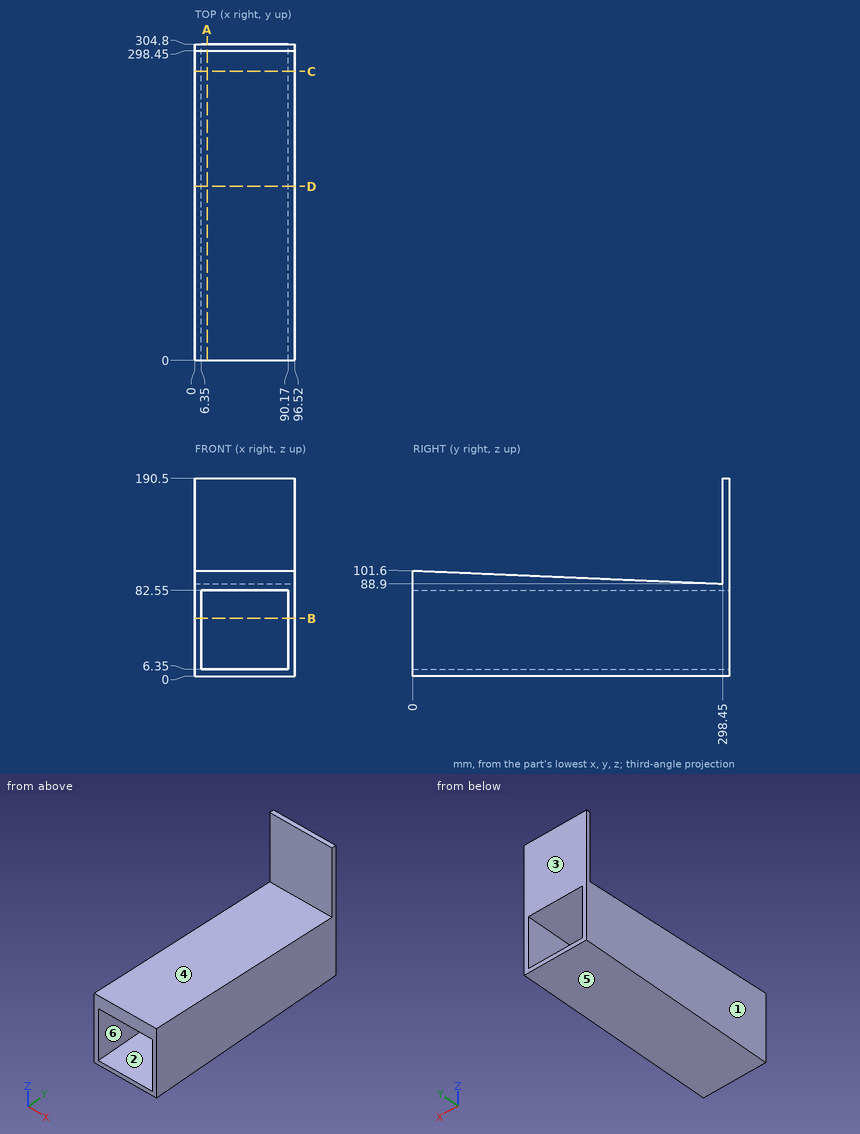
Source: three-view drawing plus pictorial views. Frame: mm from the lowest corner of the part. A direction names the side the tool comes from. Coordinates: 2 decimals unless noted, no trailing zeros. Write each loop counter-clockwise with the first axis right and the second up, starting at its lowest first coordinate (ties: lowest second). Pieces come first, ordered by that corner, then holes. Notation, with made-up numbers: (-13.5, 65) -> (12.5, 65) arc R14 ccw to (12.5, 88) -> close; hole circle Ø9 at (58.25, 32). An arc over 180 degrees is marked (long way). Write each question's results on one line, items separated by ' | '.
Item 1: Material intervals for probe 1 along X at (y, z) = (15, 62.5); probe 2 along Y at (x, z) = (29, 164); probe 3 along Z at (x, y) = (8.5, 229.5), sorted ascending.
Conclusion:
probe 1: x = 0 to 6.35, 90.17 to 96.52 | probe 2: y = 298.45 to 304.8 | probe 3: z = 0 to 6.35, 82.55 to 91.83
Item 2: Section query A-A on x = 12. Return loops of the section in (y, z), plus the area to 3 significant figures.
Conclusion:
outline: (0, 0) -> (304.8, 0) -> (304.8, 6.35) -> (0, 6.35) -> close; (0, 82.55) -> (304.8, 82.55) -> (304.8, 190.5) -> (298.45, 190.5) -> (298.45, 88.9) -> (0, 101.6) -> close | area: 6,410 mm^2
Item 3: Section query C-C on y = 278.5. Return loops of the section in (x, z), plus the area to 3 significant figures.
Conclusion:
outline: (0, 0) -> (96.52, 0) -> (96.52, 89.75) -> (0, 89.75) -> close; hole (6.35, 6.35) -> (90.17, 6.35) -> (90.17, 82.55) -> (6.35, 82.55) -> close | area: 2,280 mm^2
Item 4: Pin query (flat end, axial travel): pin 1 Ø5 at (y, z) = (122.5, 47.5) entering from -X; pin 2 Ø25 at (x, y) = (48.5, 98) entering from +Z; pin 3 Ø4 at (x, y) = (52, 70.5) entering from +Z; pin 4 Ø6 at (x, y) = (61, 49) entering from +Z. Return the tip coordinate at first contact, or that it passes through.
Conclusion:
pin 1: stops at x = 0 | pin 2: stops at z = 97.96 | pin 3: stops at z = 98.69 | pin 4: stops at z = 99.64
Item 5: Mould query, pull axis X, two halves, no side actions, for the marked faces 1, 2 and 3. Classes: +X half, -X half, draft (parallel to the pull), parting line (faces both ways), or undercut.
Conclusion:
face 1: -X half | face 2: undercut | face 3: draft
Item 6: Section query B-B on z = 55.5. Return loops of the section in (x, y), plus the area to 3 significant figures.
Conclusion:
outline: (0, 0) -> (6.35, 0) -> (6.35, 304.8) -> (0, 304.8) -> close; (90.17, 0) -> (96.52, 0) -> (96.52, 304.8) -> (90.17, 304.8) -> close | area: 3,870 mm^2
Item 7: Section query D-D on y = 167.5. Return loops of the section in (x, z), plus the area to 3 significant figures.
Conclusion:
outline: (0, 0) -> (96.52, 0) -> (96.52, 94.47) -> (0, 94.47) -> close; hole (6.35, 6.35) -> (90.17, 6.35) -> (90.17, 82.55) -> (6.35, 82.55) -> close | area: 2,730 mm^2
Item 8: Set-up query: the marked faces 4, 5 and 6. Return all of +Z, -Z, +X, -X, +Y, -Y with unobstructed straight access to the full face (end or side cutting, diameter ignored); none if empty.
Conclusion:
face 4: +Z, +X, -X | face 5: -Z, +X, -X, +Y, -Y | face 6: +Y, -Y
